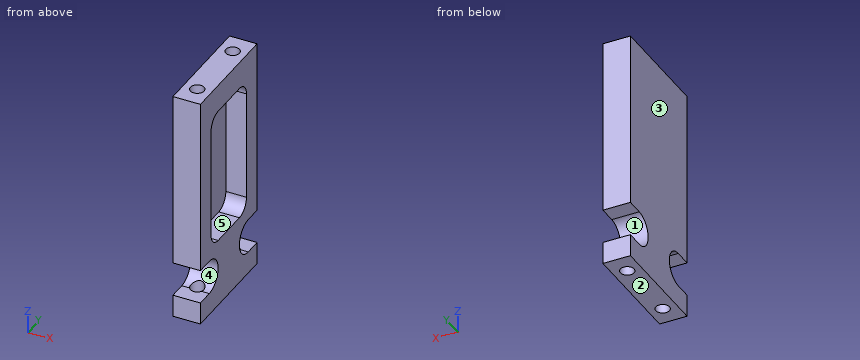
```python
from build123d import *

# Parameters (mm, degrees)
SKETCH1_W          = 107.95
SKETCH1_H          = 50.8
EXTRUDE1_DEPTH     = 12.7
SKETCH2_W          = 63.5
SKETCH2_H          = 31.75
CUT_EXTRUDE1_DEPTH = 9.525
FILLET1_R          = 6.35
CUT_EXTRUDE2_DEPTH = 120.979717036
SKETCH4_R          = 3.175
CUT_EXTRUDE3_DEPTH = 15.875
CUT_EXTRUDE4_REACH = 121.98
SKETCH5_R          = 3.175


with BuildPart() as part:
    # Sketch1 → Extrude1 (new body)
    with BuildSketch(Plane(origin=(0, 0, 0), x_dir=(0, 0, -1), z_dir=(1, 0, 0))):
        with Locations((53.975, 25.4)):
            Rectangle(SKETCH1_W, SKETCH1_H)
    extrude(amount=EXTRUDE1_DEPTH)

    # Sketch2 → Cut-Extrude1 (cut)
    with BuildSketch(Plane(origin=(12.7, 0, 0), x_dir=(0, 0, -1), z_dir=(1, 0, 0))):
        with Locations((44.45, 25.4)):
            Rectangle(SKETCH2_W, SKETCH2_H)
    extrude(amount=-CUT_EXTRUDE1_DEPTH, mode=Mode.SUBTRACT)

    # Fillet1
    fillet1_edges = [part.edges().sort_by_distance(p)[0] for p in [
        (7.9375, 9.525, -12.7),
        (7.9375, 41.275, -12.7),
        (7.9375, 41.275, -76.2),
        (7.9375, 9.525, -76.2),
    ]]
    fillet(fillet1_edges, radius=FILLET1_R)

    # Sketch3 → Cut-Extrude2 (cut, through all)
    with BuildSketch(Plane(origin=(12.7, 0, 0), x_dir=(0, 0, -1), z_dir=(1, 0, 0))):
        with BuildLine():
            Line((97.63125, 50.8), (81.75625, 50.8))
            Line((81.75625, 50.8), (81.75625, 42.8625))
            ThreePointArc((81.75625, 42.8625), (89.69375, 34.925), (97.63125, 42.8625))
            Line((97.63125, 42.8625), (97.63125, 50.8))
        make_face()
        with BuildLine():
            Line((97.63125, 0), (81.75625, 0))
            Line((81.75625, 0), (81.75625, 7.9375))
            ThreePointArc((81.75625, 7.9375), (89.69375, 15.875), (97.63125, 7.9375))
            Line((97.63125, 7.9375), (97.63125, 0))
        make_face()
    extrude(amount=-CUT_EXTRUDE2_DEPTH, mode=Mode.SUBTRACT)

    # Sketch4 → Cut-Extrude3 (cut)
    with BuildSketch(Plane.XY):
        with Locations((6.35, 41.275)):
            Circle(SKETCH4_R)
        with Locations((6.35, 9.525)):
            Circle(SKETCH4_R)
    extrude(amount=-CUT_EXTRUDE3_DEPTH, mode=Mode.SUBTRACT)

    # Sketch5 → Cut-Extrude4 (cut, up to next)
    with BuildSketch(Plane(origin=(0, 0, -107.95), x_dir=(-1, 0, 0), z_dir=(0, 0, -1)), mode=Mode.PRIVATE) as cut_extrude4_sk1:
        with Locations(Location((-6.35, 41.275, 0), (0, 0, 180))):
            Circle(SKETCH5_R)
    cut_extrude4_tool1 = extrude(cut_extrude4_sk1.sketch, amount=-CUT_EXTRUDE4_REACH, mode=Mode.PRIVATE) & part.part
    # Sketch5 → Cut-Extrude4 (cut, up to next)
    with BuildSketch(Plane(origin=(0, 0, -107.95), x_dir=(-1, 0, 0), z_dir=(0, 0, -1)), mode=Mode.PRIVATE) as cut_extrude4_sk2:
        with Locations(Location((-6.35, 9.525, 0), (0, 0, 180))):
            Circle(SKETCH5_R)
    cut_extrude4_tool2 = extrude(cut_extrude4_sk2.sketch, amount=-CUT_EXTRUDE4_REACH, mode=Mode.PRIVATE) & part.part
    add(cut_extrude4_tool1.solids().sort_by_distance((6.35, 41.275, -107.95))[0], mode=Mode.SUBTRACT)
    add(cut_extrude4_tool2.solids().sort_by_distance((6.35, 9.525, -107.95))[0], mode=Mode.SUBTRACT)


solid = part.part
```
Input: part model. Units: mm. Frame: model coordinates. Face numbers are marked on the shaded views. A direction names the side the tool comes from. Give positions to 0.01 mm unless a question says otherwise; leave off trailing zeros. Order: outer loops, then holes, each group sorted by start corner. A loop starts at its lowest first (then second) coordinate and runs counter-clockwise, first axis right, second up.
1. Draft query along Z for the marked faces 1, 2 and 3. Return one class per face: released by +Z, released by -Z, zero draft, split by the parting line, or undercut.
Computed:
face 1: undercut
face 2: released by -Z
face 3: zero draft
2. Set-up query: the marked faces 4 and 5. Return all of +Z, -Z, +X, -X, +Y, -Y with unobstructed straight access to the full face (end or side cutting, diameter ignored); none if empty.
Computed:
face 4: +X, -X, -Y
face 5: +X
3. Pin query (flat end, axial travel): pin 1 Ø1 at (y, z) = (15, -17) entering from +X (3 decimals); pin 2 Ø4 at (x, y) = (6.35, 41.275) entering from +Z (3 decimals); pin 3 Ø5 at (x, y) = (6.35, 9.525) entering from -Z. Return the tip coordinate at first contact, or that it passes through.
Computed:
pin 1: stops at x = 3.175
pin 2: stops at z = -15.875
pin 3: stops at z = -82.89
4. Cut plane C-C (z = -20.5). Return loops of the section in (x, y) (3 decimals), and give its area (3 significant figures).
Computed:
outline: (0, 0) - (12.7, 0) - (12.7, 9.525) - (3.175, 9.525) - (3.175, 41.275) - (12.7, 41.275) - (12.7, 50.8) - (0, 50.8) - close
area: 343 mm2
5. Line query: probe 1 along Y at (x, z) = (6.35, -10.5); probe 2 along Y at (x, z) = (7.5, -29.5) (3 decimals); probe 3 along Z at (x, y) = (8.5, 25). Output: solid intervals per line, ascending.
Computed:
probe 1: y = 0 to 6.35, 12.7 to 38.1, 44.45 to 50.8
probe 2: y = 0 to 9.525, 41.275 to 50.8
probe 3: z = -107.95 to -76.2, -12.7 to 0
6. Cut plane A-A (y = 24). Return loops of the section in (x, z) (3 decimals), and give its area (3 significant figures).
Computed:
outline: (0, -107.95) - (12.7, -107.95) - (12.7, -76.2) - (3.175, -76.2) - (3.175, -12.7) - (12.7, -12.7) - (12.7, 0) - (0, 0) - close
area: 766 mm2
